Design review of the part built by this model. Coordinates are the model's own, in mm. A direction names the side the tool comes from. Coordinates: 2 decimals unless noted, no trailing zeros. Order: outer loops, then holes, each group sorted by start corner. A loop starts at its lowest first (then second) coordinate and runs counter-clockwise, first axis right, second up. Notation, with made-up numbers: M 80.5,3.5 L 84.5,3.5 A26 ccw 84.5,42.5 Z; hole C -31,32.25 d6. An arc over 180 degrees is marked long. Use CSV: the item, a comma, the result in double quotes.
```python
from build123d import *

# Parameters (mm, degrees)
SKETCH_1_R                      = 10
EXTRUDE_1_DEPTH                 = 2
SKETCH_2_R                      = 4.5
EXTRUDE_2_DEPTH                 = 2.8
SKETCH_3_R                      = 3.1
CUT_EXTRUDE_1_DEPTH             = 3.8
CUT_EXTRUDE_2_REACH             = 16.644
SKETCH_4_R                      = 1.6
CUT_EXTRUDE_2_DIRECTION_2_DEPTH = 15.643770006
CUT_EXTRUDE_3_REACH             = 16.417
SKETCH_5_R                      = 1.25


with BuildPart() as part:
    # 草图1 → 凸台-拉伸1 (new body)
    with BuildSketch(Plane(origin=(0, 0, 0), x_dir=(1, 0, 0), z_dir=(0, 1, 0))):
        with Locations(Location((0, 0, 0), (0, 0, 270))):
            Circle(SKETCH_1_R)
    extrude(amount=EXTRUDE_1_DEPTH)

    # 草图2 → 凸台-拉伸2 (add)
    with BuildSketch(Plane(origin=(0, 2, 0), x_dir=(1, 0, 0), z_dir=(0, 1, 0))):
        with Locations(Location((0, 0, 0), (0, 0, 270))):
            Circle(SKETCH_2_R)
    extrude(amount=EXTRUDE_2_DEPTH)

    # 草图3 → 切除-拉伸1 (cut)
    with BuildSketch(Plane(origin=(0, 4.8, 0), x_dir=(1, 0, 0), z_dir=(0, 1, 0))):
        with Locations(Location((0, 0, 0), (0, 0, 270))):
            Circle(SKETCH_3_R)
    extrude(amount=-CUT_EXTRUDE_1_DEPTH, mode=Mode.SUBTRACT)

    # 草图4 → 切除-拉伸2 (cut, up to next)
    with BuildSketch(Plane(origin=(0, 1, 0), x_dir=(1, 0, 0), z_dir=(0, 1, 0)), mode=Mode.PRIVATE) as cut_extrude_2_sk1:
        with Locations(Location((0, 0, 0), (0, 0, 90))):
            Circle(SKETCH_4_R)
    cut_extrude_2_tool1 = extrude(cut_extrude_2_sk1.sketch, amount=-CUT_EXTRUDE_2_REACH, mode=Mode.PRIVATE) & part.part
    add(cut_extrude_2_tool1.solids().sort_by_distance((0, 1, 0))[0], mode=Mode.SUBTRACT)

    # 草图4 → 切除-拉伸2 direction 2 (cut)
    with BuildSketch(Plane(origin=(0, 1, 0), x_dir=(1, 0, 0), z_dir=(0, 1, 0))):
        with Locations(Location((0, 0, 0), (0, 0, 90))):
            Circle(SKETCH_4_R)
    extrude(amount=CUT_EXTRUDE_2_DIRECTION_2_DEPTH, mode=Mode.SUBTRACT)

    # 草图5 → 切除-拉伸3 (cut, up to next)
    with BuildSketch(Plane(origin=(0, 2, 0), x_dir=(1, 0, 0), z_dir=(0, 1, 0)), mode=Mode.PRIVATE) as cut_extrude_3_sk1:
        with Locations(Location((-7, 0, 0), (0, 0, 270))):
            Circle(SKETCH_5_R)
    cut_extrude_3_tool1 = extrude(cut_extrude_3_sk1.sketch, amount=-CUT_EXTRUDE_3_REACH, mode=Mode.PRIVATE) & part.part
    # 草图5 → 切除-拉伸3 (cut, up to next)
    with BuildSketch(Plane(origin=(0, 2, 0), x_dir=(1, 0, 0), z_dir=(0, 1, 0)), mode=Mode.PRIVATE) as cut_extrude_3_sk2:
        with Locations(Location((0, 7, 0), (0, 0, 270))):
            Circle(SKETCH_5_R)
    cut_extrude_3_tool2 = extrude(cut_extrude_3_sk2.sketch, amount=-CUT_EXTRUDE_3_REACH, mode=Mode.PRIVATE) & part.part
    # 草图5 → 切除-拉伸3 (cut, up to next)
    with BuildSketch(Plane(origin=(0, 2, 0), x_dir=(1, 0, 0), z_dir=(0, 1, 0)), mode=Mode.PRIVATE) as cut_extrude_3_sk3:
        with Locations(Location((7, 0, 0), (0, 0, 270))):
            Circle(SKETCH_5_R)
    cut_extrude_3_tool3 = extrude(cut_extrude_3_sk3.sketch, amount=-CUT_EXTRUDE_3_REACH, mode=Mode.PRIVATE) & part.part
    # 草图5 → 切除-拉伸3 (cut, up to next)
    with BuildSketch(Plane(origin=(0, 2, 0), x_dir=(1, 0, 0), z_dir=(0, 1, 0)), mode=Mode.PRIVATE) as cut_extrude_3_sk4:
        with Locations(Location((0, -7, 0), (0, 0, 270))):
            Circle(SKETCH_5_R)
    cut_extrude_3_tool4 = extrude(cut_extrude_3_sk4.sketch, amount=-CUT_EXTRUDE_3_REACH, mode=Mode.PRIVATE) & part.part
    add(cut_extrude_3_tool1.solids().sort_by_distance((-7, 2, 0))[0], mode=Mode.SUBTRACT)
    add(cut_extrude_3_tool2.solids().sort_by_distance((0, 2, -7))[0], mode=Mode.SUBTRACT)
    add(cut_extrude_3_tool3.solids().sort_by_distance((7, 2, 0))[0], mode=Mode.SUBTRACT)
    add(cut_extrude_3_tool4.solids().sort_by_distance((0, 2, 7))[0], mode=Mode.SUBTRACT)


solid = part.part
```
(1) Wall thickness on probe 1 along X at (y, z) = (1.55, 0); probe 2 along X at (y, z) = (0.6, 0); probe 3 along Y at (x, z) = (2, 6.5): over which ranges is each line inside the solid? List them lowest first.
The answers:
probe 1,"x = -10 to -8.25, -5.75 to -3.1, 3.1 to 5.75, 8.25 to 10"
probe 2,"x = -10 to -8.25, -5.75 to -1.6, 1.6 to 5.75, 8.25 to 10"
probe 3,"y = 0 to 2"
(2) Add section B-B on x = -7.5. State the section outline as (y, z) points, and give its area (3 significant figures).
The answers:
outline,"M 0,-6.61 L 2,-6.61 L 2,-1.15 L 0,-1.15 Z; M 0,1.15 L 2,1.15 L 2,6.61 L 0,6.61 Z"
area,"21.9 mm2"
(3) Add section A-A on z = 0. State the section outline as (x, y) points, and give its area (3 significant figures).
The answers:
outline,"M -10,0 L -8.25,0 L -8.25,2 L -10,2 Z; M -5.75,0 L -1.6,0 L -1.6,1 L -3.1,1 L -3.1,4.8 L -4.5,4.8 L -4.5,2 L -5.75,2 Z; M 1.6,0 L 5.75,0 L 5.75,2 L 4.5,2 L 4.5,4.8 L 3.1,4.8 L 3.1,1 L 1.6,1 Z; M 8.25,0 L 10,0 L 10,2 L 8.25,2 Z"
area,"28.4 mm2"
(4) Clearance check with flat-ended pins moving along their axes: P1, Ø2, axis at x = 0, z = 7, coming from the +Y side; P2, Ø1, axis at x = 3.5, y = 4, coming from the -Z side; P3, Ø3.5, axis at x = 0, z = 0, coming from the +Y side; P4, Ø6, axis at x = 7.5, z = -7, coming from the +Y side. State where each tip first meets the part, or that it passes through.
The answers:
P1,"passes through"
P2,"stops at z = -3.35"
P3,"stops at y = 1"
P4,"stops at y = 2"
(5) Add section C-C on y = 1.6. State the section outline as (x, z) points, and give its area (3 significant figures).
The answers:
outline,"C 0,0 d20; hole C -7,0 d2.5; hole C 0,0 d6.2; hole C 0,-7 d2.5; hole C 0,7 d2.5; hole C 7,0 d2.5"
area,"264 mm2"
(6) Add section D-D on z = -7. State the section outline as (x, y) points.
The answers:
outline,"M -7.14,0 L -1.25,0 L -1.25,2 L -7.14,2 Z; M 1.25,0 L 7.14,0 L 7.14,2 L 1.25,2 Z"
(7) For faces 5 (the face through (0.931, 2.927, 2.957)), 6 (the face through (5.78, 1.01, -0.27)), list the 3-axis set-ups (+Z, -Z, +X, -X, +Y, -Y) from which the entire face can be reached by the end or side of a thin tool; tool diameter is ignored.
The answers:
face 5,"+Y"
face 6,"+Y, -Y"
(8) The part is to be moulded in two halves that separate along Z. For faces 1 (the face through (0.05, 1.01, 5.75)), 2 (the face through (-2, 0, 0)), 3 (the face through (-8.22, 1.01, -0.27)), 4 (the face through (1.352, 3.38, 4.292)), say which applies: pulls with the +Z half, pulls with the -Z half, needs draft (parallel to the pull), parting line crosses it, or undercut.
The answers:
face 1,"undercut"
face 2,"needs draft"
face 3,"undercut"
face 4,"parting line crosses it"
